Read the model definition and answer for the solid it produces. Units are mm, in the model's axes. Face numbers are marked on the shaded views. Coordinates: 2 decimals unless noted, no trailing zeros. Write each loop counter-clockwise with the first axis right and the second up, starting at its lowest first coordinate (ties: lowest second). Pieces come first, ordered by that corner, then holes. Notation, with made-up numbers: (-1.75, 56.5) - (7.25, 56.5) arc R28 ccw to (7.25, 78.5) - close; hole circle Ø7 at (44, 82.25). An arc over 180 degrees is marked (long way). Use a Markdown table: item, result.
Autodesk Inventor part; units mm, degrees
ref_plane "YZ Plane" through (0, 0, 0) normal (1, 0, 0) x (0, 1, 0)
ref_plane "XZ Plane" through (0, 0, 0) normal (0, 1, 0) x (-1, 0, 0)
ref_plane "XY Plane" through (0, 0, 0) normal (0, 0, 1) x (1, 0, 0)
sketch "Sketch1" plane through (0, 0, 0) normal (0, 0, 1) x (1, 0, 0)
  line L0 (0, 0) -> (113, 0)
  line L1 (113, 0) -> (113, 45)
  line L2 (113, 45) -> (0, 45)
  line L3 (0, 45) -> (0, 0)
  dimension "d0" = 113
  dimension "d1" = 45
extrude "Extrusion1" add sketch "Sketch1" along normal blind 4.5
sketch "Sketch2" plane through (0, 0, 4.5) normal (0, 0, 1) x (1, 0, 0)
  circle A0 centre (56.5, 20.5) radius 7
  circle A1 centre (56.5, 20.5) radius 5
  line L0 (113, 0) -> (113, 45)
  line L1 (0, 0) -> (113, 0)
  line L2 (4.5, 38.5) -> (4.5, 6.5) construction
  circle A2 centre (4.5, 38.5) radius 2
  circle A3 centre (4.5, 22.5) radius 2
  circle A4 centre (4.5, 6.5) radius 2
  line L3 (0, 45) -> (0, 0)
  line L4 (108.5, 38.5) -> (108.5, 6.5) construction
  circle A5 centre (108.5, 38.5) radius 2
  circle A6 centre (108.5, 22.5) radius 2
  circle A7 centre (108.5, 6.5) radius 2
  line L5 (74.5, 5) -> (74.5, 21.5) construction
  circle A8 centre (74.5, 14) radius 1.5
  circle A9 centre (74.5, 5) radius 1.5
  dimension "d4" = 14
  dimension "d5" = 10
  dimension "d6" = 56.5
  dimension "d7" = 20.5
  dimension "d8" = 4
  dimension "d9" = 4
  dimension "d10" = 4
  dimension "d11" = 4.5
  dimension "d12" = 6.5
  dimension "d13" = 16
  dimension "d14" = 16
  dimension "d15" = 4
  dimension "d16" = 4
  dimension "d17" = 4
  dimension "d18" = 6.5
  dimension "d19" = 16
  dimension "d20" = 16
  dimension "d21" = 4.5
  dimension "d23" = 3
  dimension "d24" = 3
  dimension "d25" = 5
  dimension "d26" = 9
  dimension "d27" = 38.5
  dimension "d51" = 56.5
extrude "Extrusion2" add sketch "Sketch2" along normal blind 7.5 contours A0
hole "Hole1" at (56.5, 20.5, 4.5) direction (0, 0, -1) diameter 10 end through all
hole "Hole2" at (4.5, 38.5, 4.5) at (4.5, 22.5, 4.5) at (4.5, 6.5, 4.5) at (108.5, 38.5, 4.5) at (108.5, 22.5, 4.5) at (108.5, 6.5, 4.5) direction (0, 0, -1) diameter 4 end through all countersink diameter 7 countersink angle 90
hole "Hole3" at (74.5, 14, 4.5) at (74.5, 5, 4.5) direction (0, 0, -1) diameter 3 end through all
fillet "Fillet1" radius 1 4 edges at (113, 0, 2.25) (113, 45, 2.25) (0, 45, 2.25) (0, 0, 2.25)
properties part number "HUDSON 1-05-TRUCK BOLSTER PLATE"
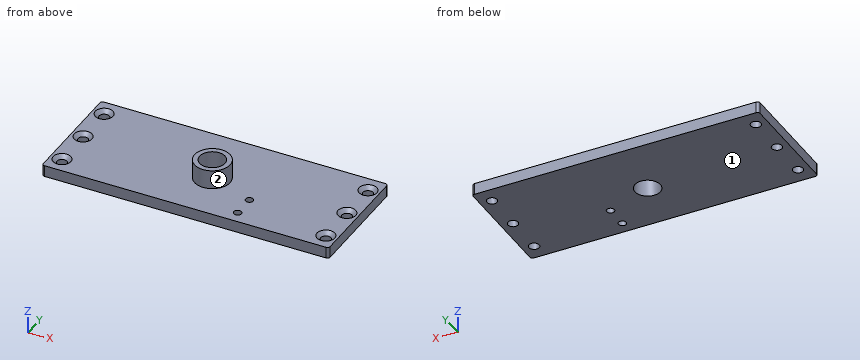
(1) A cutting plane is placed at D-D, the plane z = 6. Write down the section's boundary in (x, y).
Report:
| item | result |
|---|---|
| outline | circle Ø14 at (56.5, 20.5); hole circle Ø10 at (56.5, 20.5) |
(2) A cutting plane is placed at C-C, the plane y = 22.5. Write down the section's boundary in (x, z), and give its area (3 significant figures).
Report:
| item | result |
|---|---|
| outline | (0, 0) - (2.5, 0) - (2.5, 3) - (1, 4.5) - (0, 4.5) - close; (6.5, 0) - (51.92, 0) - (51.92, 12) - (49.79, 12) - (49.79, 4.5) - (8, 4.5) - (6.5, 3) - close; (61.08, 0) - (106.5, 0) - (106.5, 3) - (105, 4.5) - (63.21, 4.5) - (63.21, 12) - (61.08, 12) - close; (110.5, 0) - (113, 0) - (113, 4.5) - (112, 4.5) - (110.5, 3) - close |
| area | 459 mm² |
(3) The mould has two halves that part along X. Classify the marked faces 1 and 2: pulls with the +X half, pulls with the -X half, needs draft (parallel to the pull), parting line crosses it, or undercut.
Report:
| item | result |
|---|---|
| face 1 | needs draft |
| face 2 | parting line crosses it |
(4) A cutting plane is placed at A-A, the plane x = 74.5. Write down the section's boundary in (y, z), and give its area (4 significant figures).
Report:
| item | result |
|---|---|
| outline | (0, 0) - (3.5, 0) - (3.5, 4.5) - (0, 4.5) - close; (6.5, 0) - (12.5, 0) - (12.5, 4.5) - (6.5, 4.5) - close; (15.5, 0) - (45, 0) - (45, 4.5) - (15.5, 4.5) - close |
| area | 175.5 mm² |
(5) A cutting plane is placed at B-B, the plane y = 38.5. Write down the section's boundary in (x, z), and give its area (3 significant figures).
Report:
| item | result |
|---|---|
| outline | (0, 0) - (2.5, 0) - (2.5, 3) - (1, 4.5) - (0, 4.5) - close; (6.5, 0) - (106.5, 0) - (106.5, 3) - (105, 4.5) - (8, 4.5) - (6.5, 3) - close; (110.5, 0) - (113, 0) - (113, 4.5) - (112, 4.5) - (110.5, 3) - close |
| area | 468 mm² |
(6) Each of these flat-tipped pins is pushed along its axis until it touches: P1, Ø4, axis at x = 52, z = 10, coming from the +Y side; P2, Ø3, axis at x = 108.5, y = 22.5, coming from the -Z side; P3, Ø5, axis at x = 4.5, y = 38.5, coming from the +Z side; P4, Ø4.5, axis at x = 4.5, y = 22.5, coming from the +Z side. Where does it stop, or does it pass through?
Report:
| item | result |
|---|---|
| P1 | stops at y = 27.04 |
| P2 | passes through |
| P3 | stops at z = 3.5 |
| P4 | stops at z = 3.25 |
(7) Straight lines are drawn through the part: L1, parallel to X at y = 38.5, z = 1.8; L2, parallel to Y at x = 4.5, z = 0.85; L3, parallel to Y at x = 74.5, z = 3.45. For each, find the intervals that lie inside material, in ascending order.
Report:
| item | result |
|---|---|
| L1 | x = 0 to 2.5, 6.5 to 106.5, 110.5 to 113 |
| L2 | y = 0 to 4.5, 8.5 to 20.5, 24.5 to 36.5, 40.5 to 45 |
| L3 | y = 0 to 3.5, 6.5 to 12.5, 15.5 to 45 |
